Read the model definition and answer for the solid it produces. Units are mm, in the model's axes. A direction names the side the tool comes from. Give positions to 0.01 mm unless a question says otherwise; leave off trailing zeros. Order: outer loops, then holes, each group sorted by start corner. A loop starts at its lowest first (then second) coordinate and runs counter-clockwise, first axis right, second up. Notation, with made-up numbers: (74, 83.25) -> (94, 83.25) arc R16 cw to (94, 99.25) -> close; hole circle Ø6 at (51.25, 28). An arc over 180 degrees is marked (long way). Use one line per item in the form item = value.
```python
from build123d import *

# Parameters (mm, degrees)
SKICA1_R                     = 1.5
P_IDAT_VYSUNUT_M1_DEPTH      = 3
SKICA2_R                     = 1.5
P_IDAT_VYSUNUT_M2_DEPTH      = 13
P_IDAT_VYSUNUT_M2_DEPTH_BACK = 3
SKICA3_W                     = 6.5
SKICA3_H                     = 3
P_IDAT_VYSUNUT_M3_DEPTH      = 2
SKICA4_R                     = 1.35
ODEBRAT_VYSUNUT_M1_DEPTH     = 3
ZKOSEN_1_SIZE                = 1


with BuildPart() as part:
    # Skica1 → Přidat vysunutím1 (new body)
    with BuildSketch(Plane.XY):
        Polygon((0, 0), (0, 48), (16, 48), (38.5, 3), (45, 3), (45, 0), (40, 0), align=None)
        with Locations((12.9, 45.1)):
            Circle(SKICA1_R, mode=Mode.SUBTRACT)
        with Locations((2.5, 22.9)):
            Circle(SKICA1_R, mode=Mode.SUBTRACT)
        Polygon((3, 3), (35.145898034, 3), (15.37827124, 42.535253588), (3, 18), align=None, mode=Mode.SUBTRACT)
    extrude(amount=P_IDAT_VYSUNUT_M1_DEPTH)

    # Skica2 → Přidat vysunutím2 (add, two sides)
    with BuildSketch(Plane(origin=(0, 0, 0), x_dir=(-1, 0, 0), z_dir=(0, 0, -1))) as p_idat_vysunut_m2_sk:
        with Locations((-12.9, 45.1)):
            Circle(SKICA2_R)
        with Locations((-2.5, 22.9)):
            Circle(SKICA2_R)
    extrude(amount=P_IDAT_VYSUNUT_M2_DEPTH)
    extrude(p_idat_vysunut_m2_sk.sketch, amount=-P_IDAT_VYSUNUT_M2_DEPTH_BACK)

    # Skica3 → Přidat vysunutím3 (add)
    with BuildSketch(Plane.XY.offset(3)):
        with Locations((41.75, 1.5)):
            Rectangle(SKICA3_W, SKICA3_H)
    extrude(amount=P_IDAT_VYSUNUT_M3_DEPTH)

    # Skica4 → Odebrat vysunutím1 (cut)
    with BuildSketch(Plane(origin=(0, 3, 0), x_dir=(1, 0, 0), z_dir=(0, 1, 0))):
        with Locations((41.75, -2.5)):
            Circle(SKICA4_R)
    extrude(amount=-ODEBRAT_VYSUNUT_M1_DEPTH, mode=Mode.SUBTRACT)

    # Zkosení1
    zkosen_1_edges = [part.edges().sort_by_distance(p)[0] for p in [
        (40.4, 3, 2.5),
    ]]
    chamfer(zkosen_1_edges, length=ZKOSEN_1_SIZE)


solid = part.part
```
Item 1: Given pin 1 Ø5.5 at (x, z) = (42.5, 2) entering from +Y; pin 2 Ø1 at (y, z) = (41.5, -10.5) entering from +X; pin 3 Ø4 at (x, y) = (5, 31.5) entering from -Z; pin 4 Ø8 at (y, z) = (25, -9) entering from -X, each flat-ended and moving along its own axis, determine where each tip first touches the part or whether it passes through.
Checks:
pin_1 = 3
pin_2 = through
pin_3 = 0
pin_4 = 1
Item 2: The part is cut by section C-C on y = 45.1. Give the vertices of the cut face in (x, z).
Checks:
outline = (0, 0) -> (11.4, 0) -> (11.4, -13) -> (14.4, -13) -> (14.4, 0) -> (17.45, 0) -> (17.45, 3) -> (0, 3) -> close
Item 3: The part is cut by section A-A on y = 31.5. Give the vertices of the cut face in (x, z).
Checks:
outline = (0, 0) -> (9.81, 0) -> (9.81, 3) -> (0, 3) -> close; (20.9, 0) -> (24.25, 0) -> (24.25, 3) -> (20.9, 3) -> close
Item 4: Determine the mould class of faces 4 (the cylindrical face through (40.4, 1.01, 2.44)), 5 (the cylindrical face through (13.095, 46.587, -6.409)), 6 (the flat face through (3, 23, -13)) for opening direction Z: +Z half, -Z half, draft (parallel to the pull), parting line (faces both ways), or undercut.
Checks:
face_4 = undercut
face_5 = draft
face_6 = -Z half
Item 5: Straight lines are drawn through the part: L1, parallel to Z at x = 41.75, y = 1.4; L2, parallel to X at y = 1, z = 2.5; L3, parallel to X at y = 35.5, z = 1. For each, find the intervals that lie inside material, in ascending order. Write a range as from..to.
Checks:
L1 = 0..1.15, 3.85..5
L2 = 0..40.4, 43.1..45
L3 = 0..11.83, 18.9..22.25
Item 6: Which of the six approach directions +Z, -Z, +X, -X, +Y, -Y give full straight-line access (tool end or side, diameter ignored) to faces 1 (the cylindrical face through (2.825, 21.436, -6.409)), 2 (the flat face through (44, 3, 1)), 3 (the flat face through (3, 11, 1))?
Checks:
face_1 = -Z
face_2 = +Z, -Z, +X, +Y
face_3 = +Z, -Z
Item 7: The part is cut by section B-B on x = 17.5. Give the vertices of the cut face in (y, z), and give its area (3 significant figures).
Checks:
outline = (0, 0) -> (3, 0) -> (3, 3) -> (0, 3) -> close; (38.29, 0) -> (45, 0) -> (45, 3) -> (38.29, 3) -> close
area = 29.1 mm²
Item 8: The part is cut by section D-D on z = -2.5. Give the vertices of the cut face in (x, y), and give its area (3 significant figures).
Checks:
outline = circle Ø3 at (2.5, 22.9); circle Ø3 at (12.9, 45.1)
area = 14.1 mm²
